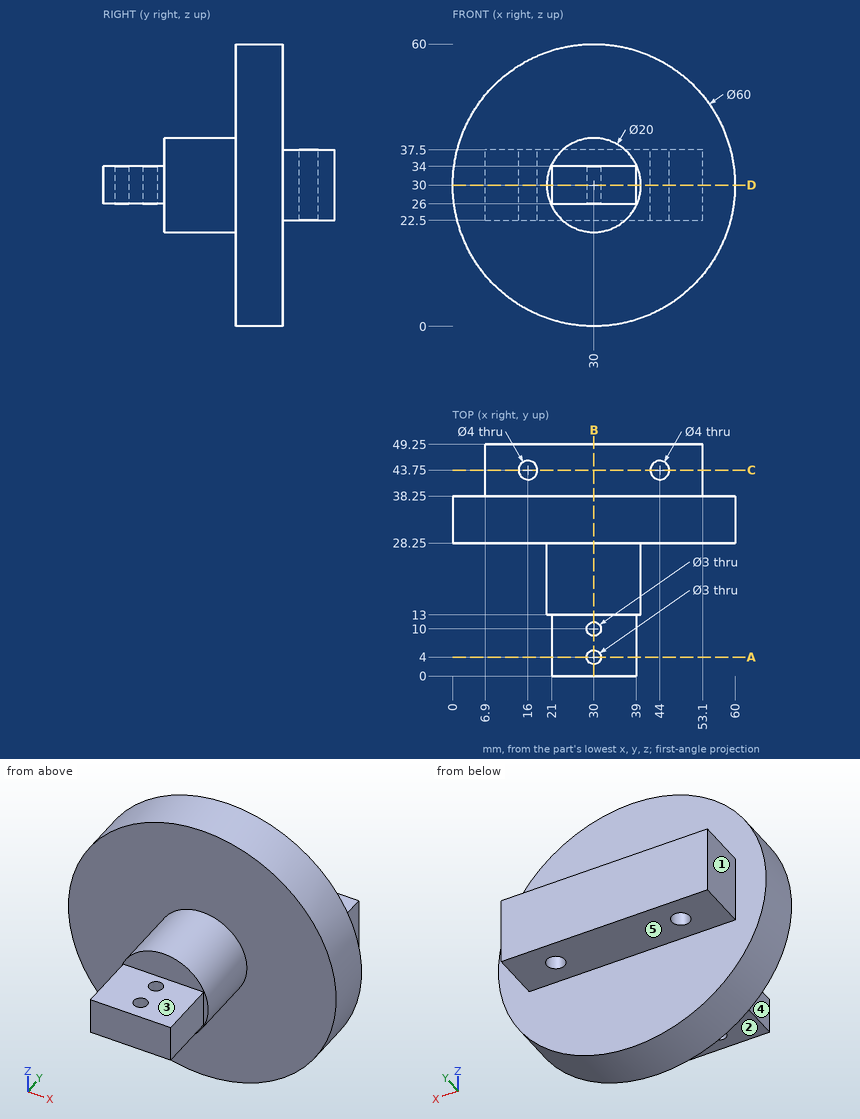
Could you check a few things on this drawing? It's one solid part, dimensions in mm from its lowest x, y, z. A direction names the side the tool comes from. Coordinates: 2 decimals unless noted, no trailing zeros. Write each loop counter-clockwise with the first axis right and the second up, starting at its lowest first coordinate (ties: lowest second). Pieces come first, ordered by that corner, then holes. Notation, with made-up numbers: (16.25, 15.5) - (48.25, 15.5) arc R19 cw to (48.25, 22.5) - close; hole circle Ø1 at (-29.5, -39.75). An arc over 180 degrees is marked (long way). Use one line per item in the form item = value.
1) I need wall thicknesses on line 1 (Y direction, x = 30, z = 31); line 2 (Y direction, x = 51, z = 20.5); line 3 (Z direction, x = 35.5, y = 10). Which ranges of each line are inside material? Lowest first, please.
Solved:
line_1 = 0 to 2.5, 5.5 to 8.5, 11.5 to 49.25
line_2 = 28.25 to 38.25
line_3 = 26 to 34
2) I'm going to push flat-ended pins straight in: P1, Ø1, axis at x = 25.5, z = 13, coming from the +Y side; P2, Ø1.5, axis at x = 18.5, y = 41, coming from the +Z side; P3, Ø4, axis at y = 18.5, z = 40.5, coming from the -X side. Where does each tip first touch, or does it pass through?
Solved:
P1 = 38.25
P2 = 37.5
P3 = 24.73
3) Suppose I cut it at D-D, the plane z = 30. Write out the boundary of the cut face in (x, y).
Solved:
outline = (0, 28.25) - (20, 28.25) - (20, 13) - (21, 13) - (21, 0) - (39, 0) - (39, 13) - (40, 13) - (40, 28.25) - (60, 28.25) - (60, 38.25) - (53.1, 38.25) - (53.1, 49.25) - (6.9, 49.25) - (6.9, 38.25) - (0, 38.25) - close; hole circle Ø4 at (16, 43.75); hole circle Ø3 at (30, 4); hole circle Ø3 at (30, 10); hole circle Ø4 at (44, 43.75)
4) Suppose I cut it at C-C, the plane y = 43.75. Write out the boundary of the cut face in (x, z).
Solved:
outline = (6.9, 22.5) - (14, 22.5) - (14, 37.5) - (6.9, 37.5) - close; (18, 22.5) - (42, 22.5) - (42, 37.5) - (18, 37.5) - close; (46, 22.5) - (53.1, 22.5) - (53.1, 37.5) - (46, 37.5) - close
5) Suppose I cut it at A-A, the plane y = 4. Write out the boundary of the cut face in (x, z).
Solved:
outline = (21, 26) - (28.5, 26) - (28.5, 34) - (21, 34) - close; (31.5, 26) - (39, 26) - (39, 34) - (31.5, 34) - close
6) On a 3-axis mill with a long thin cutter (end or side, diameter ignored), from which of +Z, -Z, +X, -X, +Y, -Y can I reach the whole of each face in a straight line? I mean the marked faces 1, 2, 3, 4 and 5. Say none if no direction works.
Solved:
face_1 = +Z, -Z, -X, +Y
face_2 = -Z, +X, -X, -Y
face_3 = +Z, +X, -X, -Y
face_4 = +Z, -Z, -X, -Y
face_5 = -Z, +X, -X, +Y
7) Suppose I cut it at B-B, the plane x = 30. Write out the boundary of the cut face in (y, z).
Solved:
outline = (0, 26) - (2.5, 26) - (2.5, 34) - (0, 34) - close; (5.5, 26) - (8.5, 26) - (8.5, 34) - (5.5, 34) - close; (11.5, 26) - (13, 26) - (13, 20) - (28.25, 20) - (28.25, 0) - (38.25, 0) - (38.25, 22.5) - (49.25, 22.5) - (49.25, 37.5) - (38.25, 37.5) - (38.25, 60) - (28.25, 60) - (28.25, 40) - (13, 40) - (13, 34) - (11.5, 34) - close
